```python
from build123d import *

# Parameters (mm, degrees)
EXTRUDE_5_DEPTH          = 3
EXTRUDE_5_DEPTH_BACK     = 1
SKETCH_1_R               = 1.6
SKETCH_6_W               = 7
SKETCH_6_H               = 9
EXTRUDE_6_DEPTH          = 10
CUT_EXTRUDE_3_DEPTH      = 48.647140523
CUT_EXTRUDE_3_DEPTH_BACK = 48.647140523
SKETCH_7_R               = 1.6
FILLET_1_R               = 2
EXTRUDE_START            = 5
EXTRUDE_7_DEPTH          = 5
SKETCH_9_R               = 3
CUT_EXTRUDE_4_DEPTH      = 3
CUT_EXTRUDE_START        = -3
SKETCH_10_R              = 3
CUT_EXTRUDE_5_DEPTH      = 3
SKETCH_11_W              = 41
SKETCH_11_H              = 3.8
EXTRUDE_8_DEPTH          = 10
FILLET_2_R               = 2


with BuildPart() as part:
    # 草图1 → 凸台-拉伸5 (new, two sides: drawn at the far end of the back side and taken through both)
    with BuildSketch(Plane.XY.offset(-EXTRUDE_5_DEPTH_BACK)):
        with BuildLine():
            Line((-11.5, -13.5), (-11.5, 11.5))
            Line((-11.5, 11.5), (-18.5, 11.5))
            ThreePointArc((-18.5, 11.5), (-19.914213562, 10.914213562), (-20.5, 9.5))
            Line((-20.5, 9.5), (-20.5, -18.5))
            ThreePointArc((-20.5, -18.5), (-19.914213562, -19.914213562), (-18.5, -20.5))
            Line((-18.5, -20.5), (18.5, -20.5))
            ThreePointArc((18.5, -20.5), (19.914213562, -19.914213562), (20.5, -18.5))
            Line((20.5, -18.5), (20.5, 9.5))
            ThreePointArc((20.5, 9.5), (19.914213562, 10.914213562), (18.5, 11.5))
            Line((18.5, 11.5), (11.5, 11.5))
            Line((11.5, 11.5), (11.5, -13.5))
            Line((11.5, -13.5), (-11.5, -13.5))
        make_face()
        with Locations((-15, 8.5)):
            Circle(SKETCH_1_R, mode=Mode.SUBTRACT)
        with Locations((-15, -8.5)):
            Circle(SKETCH_1_R, mode=Mode.SUBTRACT)
        with Locations((15, 8.5)):
            Circle(SKETCH_1_R, mode=Mode.SUBTRACT)
        with Locations((15, -8.5)):
            Circle(SKETCH_1_R, mode=Mode.SUBTRACT)
    extrude(amount=EXTRUDE_5_DEPTH + EXTRUDE_5_DEPTH_BACK)

    # 草图6 → 凸台-拉伸6 (add)
    with BuildSketch(Plane.XY.offset(3)):
        with Locations((-15, 0)):
            Rectangle(SKETCH_6_W, SKETCH_6_H)
        with Locations((15, 0)):
            Rectangle(SKETCH_6_W, SKETCH_6_H)
    extrude(amount=EXTRUDE_6_DEPTH)

    # 草图7 → 切除-拉伸3 (cut, two sides: drawn at the far end of the back side and taken through both)
    with BuildSketch(Plane.ZY.offset(20.5).offset(-CUT_EXTRUDE_3_DEPTH_BACK)):
        with Locations((9, 0)):
            Circle(SKETCH_7_R)
    extrude(amount=CUT_EXTRUDE_3_DEPTH + CUT_EXTRUDE_3_DEPTH_BACK, mode=Mode.SUBTRACT)

    # 圆角1
    fillet_1_edges = [part.edges().sort_by_distance(p)[0] for p in [
        (-11.5, -13.5, 1),
        (11.5, -13.5, 1),
    ]]
    fillet(fillet_1_edges, radius=FILLET_1_R)

    # 草图8 → 凸台-拉伸7 (add)
    with BuildSketch(Plane(origin=(0, 0, -1), x_dir=(-1, 0, 0), z_dir=(0, 0, -1)).offset(EXTRUDE_START)):
        with BuildLine():
            Line((-20.5, -18.5), (-20.5, -13.7))
            Line((-20.5, -13.7), (20.5, -13.7))
            Line((20.5, -13.7), (20.5, -18.5))
            ThreePointArc((20.5, -18.5), (19.914213562, -19.914213562), (18.5, -20.5))
            Line((18.5, -20.5), (-18.5, -20.5))
            ThreePointArc((-18.5, -20.5), (-19.914213562, -19.914213562), (-20.5, -18.5))
        make_face()
    extrude(amount=-EXTRUDE_7_DEPTH)

    # 草图9 → 切除-拉伸4 (cut)
    with BuildSketch(Plane.ZY.offset(-11.5)):
        with Locations(Location((9, 0, 0), (0, 0, 270))):
            Circle(SKETCH_9_R)
    extrude(amount=-CUT_EXTRUDE_4_DEPTH, mode=Mode.SUBTRACT)

    # 草图10 → 切除-拉伸5 (cut)
    with BuildSketch(Plane(origin=(-11.5, 0, 0), x_dir=(0, 0, -1), z_dir=(1, 0, 0)).offset(CUT_EXTRUDE_START)):
        with Locations(Location((-9, 0, 0), (0, 0, 270))):
            Circle(SKETCH_10_R)
    extrude(amount=CUT_EXTRUDE_5_DEPTH, mode=Mode.SUBTRACT)

    # 草图11 → 凸台-拉伸8 (add)
    with BuildSketch(Plane.XY.offset(3)):
        with Locations((0, -18.6)):
            Rectangle(SKETCH_11_W, SKETCH_11_H)
    extrude(amount=EXTRUDE_8_DEPTH)

    # 圆角2
    fillet_2_edges = [part.edges().sort_by_distance(p)[0] for p in [
        (-20.5, -20.5, 8),
        (20.5, -20.5, 8),
    ]]
    fillet(fillet_2_edges, radius=FILLET_2_R)


solid = part.part
```
Check sheet for the modelled part. Datum: model origin and axes. Units: mm. A direction names the side the tool comes from. Round coordinates to 2 decimals unless told otherwise and drop trailing zeros. Loops run counter-clockwise (first coordinate to the right, second up) from the corner with the lowest first, then second, coordinate; pieces in that order, holes last. Notation, with made-up numbers: (-12.5, 57.25) - (-2.5, 57.25) arc R22 cw to (-2.5, 83.25) - close; hole circle Ø9 at (63.5, -37.75). An arc over 180 degrees is marked (long way). Write item = value, one per line. Start each with the question number.
Q1. Section check C-C (z = 3.5). Record the boundary of the cut face in (x, y).
Q2. Access from +Z, -Z, +X, -X, +Y, -Y to the whole of each face (thin tool, end or side, straight path). Record for faces 4 (the face through (13, -1, -1)), 5 (the face through (0, -16.7, 8)), 6 (the face through (15, 4.5, 8)), 7 (the face through (-10.93, -12.9, 1.03)), 8 (the face through (-13, 0, 6)).
Q3. Section check D-D (y = 5.5). Record the boundary of the cut face in (x, z), plus the area to 3 significant figures.
Q4. Section check B-B (y = 0). Record the boundary of the cut face in (x, z).
Q5. Thickness scan on L1, parallel to Y at x = 15, z = 1.9; L2, parallel to Y at x = -13.8, z = 9; L3, parallel to X at y = -4, z = 2.25. Record the ranges inside material, lowest first.
Q6. Depth check by flat-ended pin: P1, Ø1, axis at y = 0.5, z = 6, coming from the -X side; P2, Ø7.5, axis at x = 9, y = 0.5, coming from the -Z side; P3, Ø3, axis at x = 2, z = 1.5, coming from the +Y side. Enter the tip coordinate at first touch or a pass-through.
Q7. Section check A-A (x = 15). Record the boundary of the cut face in (y, z).
Q8. Release check for a two-part mould opening along Y. For faces 1 (the face through (19.9, -19.93, 8.07)), 2 (the face through (12.98, -2.86, 9.9)), 3 (the face through (-15, 0, 13)) record: pulls with the +Y half, pulls with the -Y half, needs draft (parallel to the pull), parting line crosses it, or undercut.
Derived:
q1.outline = (-20.5, -18.5) arc R2 ccw to (-18.5, -20.5) - (18.5, -20.5) arc R2 ccw to (20.5, -18.5) - (20.5, -16.7) - (-20.5, -16.7) - close; (-18.5, -4.5) - (-11.5, -4.5) - (-11.5, 4.5) - (-18.5, 4.5) - close; (11.5, -4.5) - (18.5, -4.5) - (18.5, 4.5) - (11.5, 4.5) - close
q2.face_4 = -Z, +X, -X, +Y
q2.face_5 = +Z, +X, -X
q2.face_6 = +Z, +X, -X, +Y
q2.face_7 = +Z, -Z, +Y
q2.face_8 = none
q3.outline = (-20.5, -1) - (-11.5, -1) - (-11.5, 3) - (-20.5, 3) - close; (11.5, -1) - (20.5, -1) - (20.5, 3) - (11.5, 3) - close
q3.area = 72.0 mm^2
q4.outline = (-20.5, -1) - (-11.5, -1) - (-11.5, 6) - (-14.5, 6) - (-14.5, 7.4) - (-18.5, 7.4) - (-18.5, 3) - (-20.5, 3) - close; (-18.5, 10.6) - (-14.5, 10.6) - (-14.5, 12) - (-11.5, 12) - (-11.5, 13) - (-18.5, 13) - close; (11.5, -1) - (20.5, -1) - (20.5, 3) - (18.5, 3) - (18.5, 7.4) - (14.5, 7.4) - (14.5, 6) - (11.5, 6) - close; (11.5, 12) - (14.5, 12) - (14.5, 10.6) - (18.5, 10.6) - (18.5, 13) - (11.5, 13) - close
q5.L1 = -20.5 to -10.1, -6.9 to 6.9, 10.1 to 11.5
q5.L2 = -20.5 to -16.7, -4.5 to -3, 3 to 4.5
q5.L3 = -20.5 to -11.5, 11.5 to 20.5
q6.P1 = -18.5
q6.P2 = -1
q6.P3 = -13.5
q7.outline = (-20.5, -6) - (-13.7, -6) - (-13.7, -1) - (-10.1, -1) - (-10.1, 3) - (-16.7, 3) - (-16.7, 13) - (-20.5, 13) - close; (-6.9, -1) - (6.9, -1) - (6.9, 3) - (4.5, 3) - (4.5, 13) - (-4.5, 13) - (-4.5, 3) - (-6.9, 3) - close; (10.1, -1) - (11.5, -1) - (11.5, 3) - (10.1, 3) - close; hole circle Ø3.2 at (0, 9)
q8.face_1 = pulls with the -Y half
q8.face_2 = undercut
q8.face_3 = needs draft
